Input: part model. Units: mm. Frame: model coordinates. A direction names the side the tool comes from. Coordinates: 2 decimals unless noted, no trailing zeros. Loops run counter-clockwise (first coordinate to the right, second up) from the corner with the lowest first, then second, coordinate; pieces in that order, holes last. Notation, with made-up numbers: (-15, 36.25) -> (35, 36.25) arc R25 cw to (35, 57.25) -> close; hole circle Ø7 at (59, 17). An arc over 180 degrees is marked (long way). Answer as a JSON object with one key per item and string values.
from build123d import *

# Parameters (mm, degrees)
SKETCH1_R                  = 3.7
SKETCH1_R_2                = 2.4
PIN_SIDE_DEPTH             = 3.7
SIDE_START                 = 3.7
SIDE_EAR_DEPTH             = 1
MIDDLE_RIB_DEPTH           = 0.7
SKETCH4_R                  = 2.85
AXLE_BODY_DEPTH            = 3.7
AXLE_CUT_DEPTH             = 21.383081219
AXLE_CUT_DEPTH_BACK        = 21.383081219
SKETCH5_W                  = 1.8
SKETCH5_H                  = 1.8
AXLE_SLOT_DEPTH            = 21.383081219
AXLE_SLOT_DEPTH_BACK       = 21.383081219
SKETCH8_R                  = 3.7
SKETCH8_R_2                = 2.4
SECOND_PIN_BODY_DEPTH      = 3.7
SECOND_PIN_HOLE_DEPTH      = 21.383081238
SECOND_PIN_HOLE_DEPTH_BACK = 21.383081238
SKETCH9_R                  = 2.4
SKETCH7_R                  = 3.1
PIN_RIM_DEPTH              = 0.8
FILLET1_R                  = 0.5
MIRROR2_START              = -3.7
MIRROR2_OUTLINE_R          = 3.1
MIRROR2_OUTLINE_R_2        = 2.4
MIRROR2_DEPTH              = 0.8
MIRROR2_2_DEPTH            = 3
MIRROR2_START_2            = 0.7
MIRROR2_3_DEPTH            = 3


# Read off the part's stored shape, not the designer's step: Mirror2
with BuildPart() as part:
    # Sketch1 → Pin Side (new, symmetric)
    with BuildSketch(Plane.XY):
        Circle(SKETCH1_R)
        Circle(SKETCH1_R_2, mode=Mode.SUBTRACT)
    extrude(amount=PIN_SIDE_DEPTH, both=True)

    # Sketch2 → Side Ear (add)
    with BuildSketch(Plane(origin=(0, 0, 0), x_dir=(1, 0, 0), z_dir=(0, 1, 0)).offset(SIDE_START)):
        with BuildLine():
            Line((0, 3.7), (0, -3.7))
            Line((0, -3.7), (16, -3.7))
            ThreePointArc((16, -3.7), (19.7, 0), (16, 3.7))
            Line((16, 3.7), (0, 3.7))
        make_face()
    side_ear = extrude(amount=-SIDE_EAR_DEPTH)

    # Mirror1: Side Ear across plane
    add(side_ear.mirror(Plane.ZX))

    # Sketch3 → Middle Rib (add, symmetric)
    with BuildSketch(Plane.XY):
        with BuildLine():
            Line((2.529822128, -2.7), (16, -2.7))
            Line((16, -2.7), (16, 2.7))
            Line((16, 2.7), (2.529822128, 2.7))
            ThreePointArc((2.529822128, 2.7), (3.7, 0), (2.529822128, -2.7))
        make_face()
    extrude(amount=MIDDLE_RIB_DEPTH, both=True)

    # Sketch4 → Axle Body (add, symmetric)
    with BuildSketch(Plane(origin=(0, 0, 0), x_dir=(1, 0, 0), z_dir=(0, 1, 0))):
        with Locations((16, 0)):
            Circle(SKETCH4_R)
    extrude(amount=AXLE_BODY_DEPTH, both=True)

    # Sketch5 → Axle Cut (cut, two sides: drawn at the far end of the back side and taken through both)
    with BuildSketch(Plane(origin=(0, 0, 0), x_dir=(1, 0, 0), z_dir=(0, 1, 0)).offset(-AXLE_CUT_DEPTH_BACK)):
        with BuildLine():
            Line((13.775140454, -0.9), (15.1, -0.9))
            Line((15.1, -0.9), (15.1, 0.9))
            Line((15.1, 0.9), (13.775140454, 0.9))
            ThreePointArc((13.775140454, 0.9), (13.644191974, 0.45844143), (13.6, 0))
            ThreePointArc((13.6, 0), (13.644191974, -0.45844143), (13.775140454, -0.9))
        make_face()
        with BuildLine():
            Line((15.1, 0.9), (16.9, 0.9))
            Line((16.9, 0.9), (16.9, 2.224859546))
            ThreePointArc((16.9, 2.224859546), (16.45844143, 2.355808026), (16, 2.4))
            ThreePointArc((16, 2.4), (15.54155857, 2.355808026), (15.1, 2.224859546))
            Line((15.1, 2.224859546), (15.1, 0.9))
        make_face()
        with Locations((16, 0)):
            Rectangle(SKETCH5_W, SKETCH5_H)
        with BuildLine():
            Line((16.9, 0.9), (16.9, -0.9))
            Line((16.9, -0.9), (18.224859546, -0.9))
            ThreePointArc((18.224859546, -0.9), (18.355808026, -0.45844143), (18.4, 0))
            ThreePointArc((18.4, 0), (18.355808026, 0.45844143), (18.224859546, 0.9))
            Line((18.224859546, 0.9), (16.9, 0.9))
        make_face()
        with BuildLine():
            ThreePointArc((15.1, -2.224859546), (15.54155857, -2.355808026), (16, -2.4))
            ThreePointArc((16, -2.4), (16.45844143, -2.355808026), (16.9, -2.224859546))
            Line((16.9, -2.224859546), (16.9, -0.9))
            Line((16.9, -0.9), (15.1, -0.9))
            Line((15.1, -0.9), (15.1, -2.224859546))
        make_face()
    extrude(amount=AXLE_CUT_DEPTH + AXLE_CUT_DEPTH_BACK, mode=Mode.SUBTRACT)

    # Sketch6 → Axle Slot (cut, two sides: drawn at the far end of the back side and taken through both)
    with BuildSketch(Plane.XY.offset(-AXLE_SLOT_DEPTH_BACK)):
        with BuildLine():
            Line((15.5, -2.2), (15.5, 2.2))
            ThreePointArc((15.5, 2.2), (16, 2.7), (16.5, 2.2))
            Line((16.5, 2.2), (16.5, -2.2))
            ThreePointArc((16.5, -2.2), (16, -2.7), (15.5, -2.2))
        make_face()
    extrude(amount=AXLE_SLOT_DEPTH + AXLE_SLOT_DEPTH_BACK, mode=Mode.SUBTRACT)

    # Sketch8 → Second Pin Body (add, symmetric)
    with BuildSketch(Plane.XY):
        with Locations((8, 0)):
            Circle(SKETCH8_R)
        with Locations((8, 0)):
            Circle(SKETCH8_R_2, mode=Mode.SUBTRACT)
    extrude(amount=SECOND_PIN_BODY_DEPTH, both=True)

    # Sketch9 → Second Pin Hole (cut, two sides: drawn at the far end of the back side and taken through both)
    with BuildSketch(Plane.XY.offset(-SECOND_PIN_HOLE_DEPTH_BACK)):
        with Locations((8, 0)):
            Circle(SKETCH9_R)
    extrude(amount=SECOND_PIN_HOLE_DEPTH + SECOND_PIN_HOLE_DEPTH_BACK, mode=Mode.SUBTRACT)

    # Sketch7 → Pin Rim (cut)
    with BuildSketch(Plane.XY.offset(3.7)):
        Circle(SKETCH7_R)
        with Locations((8, 0)):
            Circle(SKETCH7_R)
    extrude(amount=-PIN_RIM_DEPTH, mode=Mode.SUBTRACT)

    # Fillet1
    fillet1_edges = [part.edges().sort_by_distance(p)[0] for p in [
        (5.470177872, -2.7, 2.2),
        (5.470177872, 2.7, 2.2),
        (2.529822128, -2.7, 2.2),
        (2.529822128, 2.7, 2.2),
    ]]
    fillet(fillet1_edges, radius=FILLET1_R)

    # Mirror2 outline → Mirror2 (cut)
    # profile 1 of 2: a face of its own
    with BuildSketch(Plane.XY.offset(MIRROR2_START)):
        with Locations((8, 0)):
            Circle(MIRROR2_OUTLINE_R)
        with Locations((8, 0)):
            Circle(MIRROR2_OUTLINE_R_2, mode=Mode.SUBTRACT)
    # profile 2 of 2: a face of its own
    with BuildSketch(Plane.XY.offset(MIRROR2_START)):
        Circle(MIRROR2_OUTLINE_R)
        Circle(MIRROR2_OUTLINE_R_2, mode=Mode.SUBTRACT)
    extrude(amount=MIRROR2_DEPTH, mode=Mode.SUBTRACT)

    # Mirror2 2 outline → Mirror2 2 (add)
    with BuildSketch(Plane.XY.offset(MIRROR2_START)):
        with BuildLine():
            ThreePointArc((2.529822128, 2.7), (2.86623565, 2.33980623), (3.151791054, 1.938095238))
            ThreePointArc((3.151791054, 1.938095238), (3.141272984, 2.443975018), (3.577708764, 2.7))
            Line((3.577708764, 2.7), (2.529822128, 2.7))
        make_face()
        with BuildLine():
            ThreePointArc((3.577708764, -2.7), (3.141272984, -2.443975018), (3.151791054, -1.938095238))
            ThreePointArc((3.151791054, -1.938095238), (2.86623565, -2.33980623), (2.529822128, -2.7))
            Line((2.529822128, -2.7), (3.577708764, -2.7))
        make_face()
    extrude(amount=MIRROR2_2_DEPTH)

    # Mirror2 3 outline → Mirror2 3 (add)
    with BuildSketch(Plane.XY.offset(MIRROR2_START_2)):
        with BuildLine():
            ThreePointArc((10.529822128, 2.7), (10.86623565, 2.33980623), (11.151791054, 1.938095238))
            ThreePointArc((11.151791054, 1.938095238), (11.141272984, 2.443975018), (11.577708764, 2.7))
            Line((11.577708764, 2.7), (10.529822128, 2.7))
        make_face()
        with BuildLine():
            ThreePointArc((11.577708764, -2.7), (11.141272984, -2.443975018), (11.151791054, -1.938095238))
            ThreePointArc((11.151791054, -1.938095238), (10.86623565, -2.33980623), (10.529822128, -2.7))
            Line((10.529822128, -2.7), (11.577708764, -2.7))
        make_face()
    extrude(amount=MIRROR2_3_DEPTH)


solid = part.part
1. Pin query (flat end, axial travel): P1, Ø2, axis at x = 15.5, y = -1.5, coming from the +Z side; P2, Ø1.5, axis at y = 1, z = 1.5, coming from the +X side; P3, Ø0.7, axis at x = 14.5, y = 0, coming from the -Z side. Return the tip coordinate at first contact, or that it passes through.
Reply:
{"P1": "stops at z = 2.82", "P2": "stops at x = 18.75", "P3": "stops at z = -2.61"}
2. Mould query, pull axis Z, two halves, no side actions, for faces 6 (the face through (10, -3.7, 0)), 7 (the face through (14, 0, 0.9)), 8 (the face through (2, -2, 2.9)). Classes: pulls with the +Z half, pulls with the -Z half, needs draft (parallel to the pull), parting line crosses it, or undercut.
Reply:
{"face 6": "needs draft", "face 7": "undercut", "face 8": "pulls with the +Z half"}
3. Section query A-A (x = 8.75). Return loops of the section in (y, z).
Reply:
{"outline": "(-3.7, -3.7) -> (-3.01, -3.7) -> (-3.01, -2.9) -> (-2.28, -2.9) -> (-2.28, 2.9) -> (-3.01, 2.9) -> (-3.01, 3.7) -> (-3.7, 3.7) -> close; (2.28, -2.9) -> (3.01, -2.9) -> (3.01, -3.7) -> (3.7, -3.7) -> (3.7, 3.7) -> (3.01, 3.7) -> (3.01, 2.9) -> (2.28, 2.9) -> close"}
4. Section query C-C (y = 0). Count the separate pieces of the cut face and the enclosed holes in it, plus the area to 3 significant figures.
Reply:
{"separate pieces": "4", "enclosed holes": "0", "area": "47.9 mm2"}
5. Access query for faces 1 (the face through (-3.7, 0.1, 0.1)), 2 (the face through (13, -2.7, -1)), 3 (the face through (16.9, 0, -2)), 4 (the face through (4, 0, -0.7)), 5 (the face through (4, -2.7, 2)). Directions: +Z, -Z, +X, -X, +Y, -Y. A direction counts if a zero-diameter tool reaches every point of the face in a straight line with its end or side. Return the directions, or none.
Reply:
{"face 1": "+Z, -Z, -X", "face 2": "none", "face 3": "+Y, -Y", "face 4": "-Z", "face 5": "+Z"}
6. Section query B-B (z = -0.25). Return loops of the section in (x, y), plus the area to 3 significant figures.
Reply:
{"outline": "(0, -3.7) -> (13.61, -3.7) -> (13.61, 3.7) -> (0, 3.7) arc R3.7 ccw to start; (18.39, -3.7) -> (19.69, -3.7) -> (19.69, -2.7) -> (18.84, -2.7) -> (18.84, 2.7) -> (19.69, 2.7) -> (19.69, 3.7) -> (18.39, 3.7) -> close; hole circle Ø4.8 at (0, 0); hole circle Ø4.8 at (8, 0)", "area": "91.1 mm2"}
7. Section query D-D (x = -1.75). Return loops of the section in (y, z), plus the area to 3 significant figures.
Reply:
{"outline": "(-3.26, -3.7) -> (-2.56, -3.7) -> (-2.56, -2.9) -> (-1.64, -2.9) -> (-1.64, 2.9) -> (-2.56, 2.9) -> (-2.56, 3.7) -> (-3.26, 3.7) -> close; (1.64, -2.9) -> (2.56, -2.9) -> (2.56, -3.7) -> (3.26, -3.7) -> (3.26, 3.7) -> (2.56, 3.7) -> (2.56, 2.9) -> (1.64, 2.9) -> close", "area": "21.0 mm2"}
8. Line query: line 1 along Y through (x, z) = (8, -3.35); line 2 along Y through (x, z) = (11.75, -2); line 3 along X through (y, z) = (0, 1). Output: solid intervals per line, ascending.
Reply:
{"line 1": "y = -3.7 to -3.1, 3.1 to 3.7", "line 2": "y = -3.7 to -2.7, 2.7 to 3.7", "line 3": "x = -3.7 to -2.4, 2.4 to 3.7, 4.3 to 5.6, 10.4 to 11.7, 13.33 to 15.1, 16.9 to 18.67"}
